Can you work these out from the model? Positions are in its coordinate system, mm. Face numbers are marked on the shaded views. Round coordinates to 2 decimals unless told otherwise and drop trailing zeros. Loops run counter-clockwise (first coordinate to the right, second up) from the corner with the lowest first, then second, coordinate; pieces in that order, holes last.
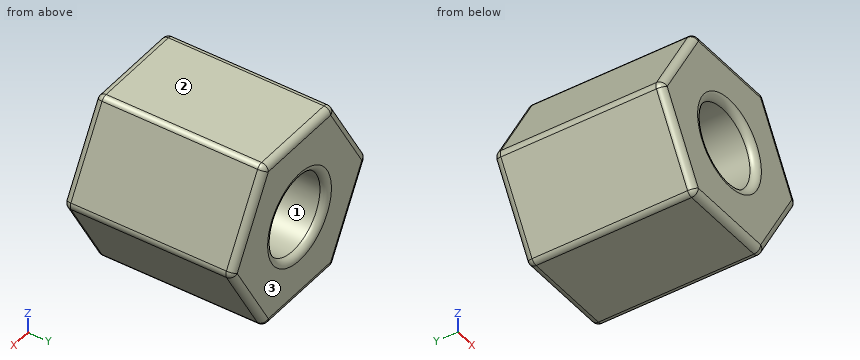
from build123d import *

# Parameters (mm, degrees)
SKETCH1_R           = 1.4732
BOSS_EXTRUDE1_DEPTH = 6.35
FILLET1_R           = 0.254


with BuildPart() as part:
    # Sketch1 → Boss-Extrude1 (new body)
    with BuildSketch(Plane(origin=(0, 0, 0), x_dir=(1, 0, 0), z_dir=(0, 1, 0))):
        Polygon((1.833087105, -3.175), (3.666174209, 0), (1.833087105, 3.175), (-1.833087105, 3.175), (-3.666174209, 0), (-1.833087105, -3.175), align=None)
        Circle(SKETCH1_R, mode=Mode.SUBTRACT)
    extrude(amount=BOSS_EXTRUDE1_DEPTH)

    # Fillet1
    fillet1_edges = [part.edges().sort_by_distance(p)[0] for p in [
        (2.749630657, 6.35, -1.5875),
        (-1.833087105, 3.175, 3.175),
        (-3.666174209, 3.175, 0),
        (-1.833087105, 3.175, -3.175),
        (1.833087105, 3.175, -3.175),
        (3.666174209, 3.175, 0),
        (1.833087105, 3.175, 3.175),
        (0, 6.35, -3.175),
        (-2.749630657, 6.35, -1.5875),
        (-1.4732, 0, 0),
        (-1.4732, 6.35, 0),
        (-2.749630657, 6.35, 1.5875),
        (0, 6.35, 3.175),
        (-2.749630657, 0, 1.5875),
        (-2.749630657, 0, -1.5875),
        (0, 0, -3.175),
        (2.749630657, 6.35, 1.5875),
        (2.749630657, 0, -1.5875),
        (2.749630657, 0, 1.5875),
        (0, 0, 3.175),
    ]]
    fillet(fillet1_edges, radius=FILLET1_R)


solid = part.part
(1) If we section it at A-A, the plane x = 0: List the corners of the cut face in (y, z) for me (3 decimals).
Worked answers:
outline: (0, -2.921) arc R0.254 ccw to (0.254, -3.175) - (6.096, -3.175) arc R0.254 ccw to (6.35, -2.921) - (6.35, -1.727) arc R0.254 ccw to (6.096, -1.473) - (0.254, -1.473) arc R0.254 ccw to (0, -1.727) - close; (0, 1.727) arc R0.254 ccw to (0.254, 1.473) - (6.096, 1.473) arc R0.254 ccw to (6.35, 1.727) - (6.35, 2.921) arc R0.254 ccw to (6.096, 3.175) - (0.254, 3.175) arc R0.254 ccw to (0, 2.921) - close
(2) If we mould it in two halves opening along Z, with no side actions, what happens to the marked faces 1, 2 and 3? For each: released by +Z, released by -Z, zero draft, split by the parting line, or undercut.
Worked answers:
face 1: undercut
face 2: released by +Z
face 3: zero draft
(3) If we section it at B-B, the plane y = 2.25: List the corners of the cut face in (x, z) for me (3 decimals), then the cut area to 3 significant figures.
Worked answers:
outline: (-3.593, -0.127) - (-1.906, -3.048) arc R0.254 ccw to (-1.686, -3.175) - (1.686, -3.175) arc R0.254 ccw to (1.906, -3.048) - (3.593, -0.127) arc R0.254 ccw to (3.593, 0.127) - (1.906, 3.048) arc R0.254 ccw to (1.686, 3.175) - (-1.686, 3.175) arc R0.254 ccw to (-1.906, 3.048) - (-3.593, 0.127) arc R0.254 ccw to start; hole circle Ø2.946 at (0, 0)
area: 28.1 mm2
(4) If I drill on line 1 (Z direction, x = 0, y = 4.2) (3 decimals); line 2 (X direction, y = 3.7, z = 0); line 3 (X direction, y = 5, z = -1), over which ranges is the centre line in solid material (lowest first)?
Worked answers:
line 1: z = -3.175 to -1.473, 1.473 to 3.175
line 2: x = -3.63 to -1.47, 1.47 to 3.63
line 3: x = -3.09 to -1.08, 1.08 to 3.09
